Autodesk Inventor part; units mm, degrees
ref_plane "YZ Plane" through (0, 0, 0) normal (1, 0, 0) x (0, 1, 0)
ref_plane "XZ Plane" through (0, 0, 0) normal (0, 1, 0) x (-1, 0, 0)
ref_plane "XY Plane" through (0, 0, 0) normal (0, 0, 1) x (1, 0, 0)
sketch "スケッチ1" plane through (0, 0, 0) normal (0, 0, 1) x (1, 0, 0)
  circle A0 centre (0, 0) radius 47.6
  circle A1 centre (0, 0) radius 67.5
  dimension "d0" = 95.2
  dimension "d1" = 135
extrude "押し出し1" add sketch "スケッチ1" along normal blind 20
sketch "スケッチ2" plane through (0, 0, 20) normal (0, 0, 1) x (1, 0, 0)
  circle A0 centre (0, 0) radius 62.5
  point P0 (16.1762, 60.3704)
  point P1 (-16.1762, 60.3704)
  point P2 (-44.1942, 44.1942)
  point P3 (-60.3704, 16.1762)
  point P4 (-60.3704, -16.1762)
  point P5 (-44.1942, -44.1942)
  point P6 (-16.1762, -60.3704)
  point P7 (16.1762, -60.3704)
  point P8 (44.1942, -44.1942)
  point P9 (60.3704, -16.1762)
  point P10 (60.3704, 16.1762)
  point P11 (44.1942, 44.1942)
  dimension "d4" = 125
  dimension "d7" = 360
  dimension "d25" = 0
hole "穴1" at (16.1762, 60.3704, 20) at (-16.1762, 60.3704, 20) at (-44.1942, 44.1942, 20) at (-60.3704, 16.1762, 20) at (-60.3704, -16.1762, 20) at (-44.1942, -44.1942, 20) at (-16.1762, -60.3704, 20) at (16.1762, -60.3704, 20) at (44.1942, -44.1942, 20) at (60.3704, -16.1762, 20) at (60.3704, 16.1762, 20) at (44.1942, 44.1942, 20) direction (0, 0, -1) diameter 4.3 end through all
chamfer "面取り1" distance 1 angle 45 2 edges at (-47.6, 0, 20) (-47.6, 0, 0)
sketch "スケッチ3" plane through (0, 0, 20) normal (0, 0, 1) x (1, 0, 0)
  circle A0 centre (16.1762, 60.3704) radius 2.15
  circle A1 centre (-16.1762, 60.3704) radius 2.15
  circle A2 centre (0, 0) radius 67.5
  circle A3 centre (-16.1762, 60.3704) radius 5
  circle A4 centre (16.1762, 60.3704) radius 5
  circle A5 centre (0, 0) radius 62.5
  point P0 (-11.2987, 61.4702)
  point P1 (11.2987, 61.4702)
  point P2 (17.4703, 65.2)
  point P3 (-17.4703, 65.2)
properties part number "unit-base3" material "ABS プラスチック"
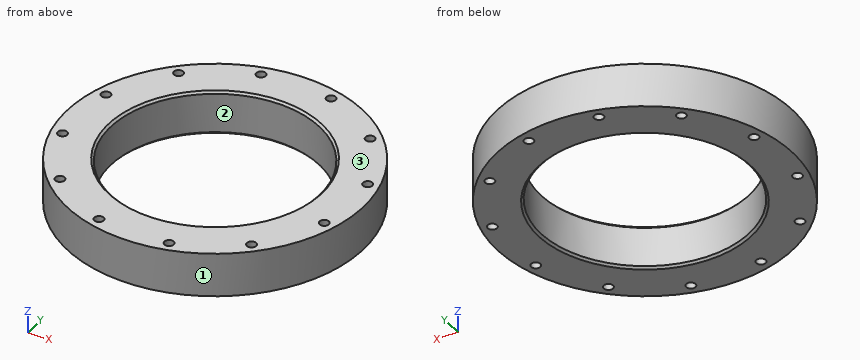
Geometry: final body of the model. Coordinates: model frame, mm. Face numbers are marked on the shaded views. Round coordinates to 2 decimals unless told otherwise and drop trailing zeros. Loops run counter-clockwise (first coordinate to the right, second up) from the corner with the lowest first, then second, coordinate; pieces in that order, holes last. Notation, with made-up numbers: (-38.75, 82) -> (-11.75, 82) arc R7 cw to (-11.75, 94) -> close; hole circle Ø3 at (49, 8.5). An arc over 180 degrees is marked (long way). Use one line per item in the form item = value.
Item 1: Material intervals for probe 1 along Y at (x, z) = (0, 8); probe 2 along X at (y, z) = (61.5, 18); probe 3 along Y at (x, z) = (-62, 11.5), sorted ascending.
Evaluation:
probe_1 = -67.5 to -47.6, 47.6 to 67.5
probe_2 = -27.82 to -18.01, -14.35 to 14.35, 18.01 to 27.82
probe_3 = -26.69 to -17.58, -14.77 to 14.77, 17.58 to 26.69
Item 2: Draft query along Y for the marked faces 1, 2 and 3. Return one class per face: released by +Y, released by -Y, zero draft, split by the parting line, or undercut.
Evaluation:
face_1 = split by the parting line
face_2 = undercut
face_3 = zero draft
Item 3: Contact query for flat-ended pins moving along their axis: pin 1 Ø12 at (x, z) = (-34, 15) entering from +Y; pin 2 Ø2 at (x, z) = (-38, 15) entering from -Y; pin 3 Ø5 at (x, z) = (-25, 8.5) entering from -Y. Output: stop coordinate, or through.
Evaluation:
pin_1 = 61.42
pin_2 = -56.46
pin_3 = -63.64
Item 4: Cut plane A-A on x = 0. Output: boundary loops of the cut face in (y, z).
Evaluation:
outline = (-67.5, 0) -> (-48.6, 0) -> (-47.6, 1) -> (-47.6, 19) -> (-48.6, 20) -> (-67.5, 20) -> close; (47.6, 1) -> (48.6, 0) -> (67.5, 0) -> (67.5, 20) -> (48.6, 20) -> (47.6, 19) -> close
Item 5: Cut plane C-C on z = 12.5. Give the number of separate pieces and of enclosed holes in the cut face, then the cut area to 3 significant figures.
Evaluation:
separate_pieces = 1
enclosed_holes = 13
area = 7,020 mm2
